```python
from build123d import *

# Parameters (mm, degrees)
F2_SIZE = 0.2


with BuildPart() as f1:
    # F0 (on Front) → F1 (revolve)
    with BuildSketch(Plane.XZ):
        Polygon((3.8, 27), (3.8, 0), (4.5, 0), (4.5, 14.8), (6.5, 14.8), (6.5, 21.4), (4.5, 21.4), (4.5, 27), align=None)
    revolve(axis=Axis((0, 0, 50), (0, 0, -1)))

    # F2
    f2_edges = [f1.edges().sort_by_distance(p)[0] for p in [
        (-4.5, 0, 0),
        (-6.5, 0, 14.8),
        (-6.5, 0, 21.4),
        (-4.5, 0, 27),
        (-3.8, 0, 27),
        (-3.8, 0, 0),
    ]]
    chamfer(f2_edges, length=F2_SIZE)


solid = f1.part
```
Part model, mm, in its own coordinate system. A direction names the side the tool comes from. Round coordinates to 2 decimals unless told otherwise and drop trailing zeros. Write each loop counter-clockwise with the first axis right and the second up, starting at its lowest first coordinate (ties: lowest second). Pieces come first, ordered by that corner, then holes. Notation, with made-up numbers: M -4,54 L 4,54 A13 ccw 4,62 Z; hole C -7,76.5 d10. An arc over 180 degrees is marked long. One line per question, with ' | ' between items.
(1) Saw through at C-C on z = 20.5. Write the cut outline in (x, y), then the cut area to 3 significant figures.
Answer key:
outline: C 0,0 d13; hole C 0,0 d7.6 | area: 87.4 mm^2
(2) Two-plate mould, pull along X, no slides. Class faces 1 (the face through (4, 3, 21.4)), 2 (the face through (-3.796, -0.167, 13.314)), 3 (the face through (-0.59, -4.46, 24.14)): released by +X, released by -X, zero draft, split by the parting line, or undercut.
Answer key:
face 1: zero draft | face 2: undercut | face 3: split by the parting line
(3) Saw through at A-A on y = 0. Write the cut outline in (x, z).
Answer key:
outline: M -6.5,15 L -6.3,14.8 L -4.5,14.8 L -4.5,0.2 L -4.3,0 L -4,0 L -3.8,0.2 L -3.8,26.8 L -4,27 L -4.3,27 L -4.5,26.8 L -4.5,21.4 L -6.3,21.4 L -6.5,21.2 Z; M 3.8,0.2 L 4,0 L 4.3,0 L 4.5,0.2 L 4.5,14.8 L 6.3,14.8 L 6.5,15 L 6.5,21.2 L 6.3,21.4 L 4.5,21.4 L 4.5,26.8 L 4.3,27 L 4,27 L 3.8,26.8 Z
(4) Probe line 1 along Y through (x, z) = (0, 8.25); line 2 along Y through (x, z) = (0, 17.25). List the from-to ranges inside material, lowest first.
Answer key:
line 1: y = -4.5 to -3.8, 3.8 to 4.5 | line 2: y = -6.5 to -3.8, 3.8 to 6.5
(5) 3-axis set-ups, long thin cutter, end or side, ignore diameter. For faces 4 (the face through (-5.158, 3.955, 18.143)), 5 (the face through (-4, 3, 14.8)): which of +Z, -Z, +X, -X, +Y, -Y reach the whole face in a straight line?
Answer key:
face 4: +Z, -Z | face 5: -Z
(6) Saw through at D-D on z = 3. Write the cut outline in (x, y), then the cut area to 3 significant figures.
Answer key:
outline: C 0,0 d9; hole C 0,0 d7.6 | area: 18.3 mm^2
(7) Pin check, flat tips, straight feed: pin 1 (6 mm diameter, centred on x = -1, z = 9.5, fed in from -Y); pin 2 (6 mm diameter, centred on x = 5, z = 14, fed in from -Y); pin 3 (4 mm diameter, centred on x = -1, z = 10.5, fed in from +Y); pin 4 (6.5 mm diameter, centred on x = 2, y = 3, fed in from +Z). Stop position of each tip, or through.
Answer key:
pin 1: stops at y = -4.5 | pin 2: stops at y = -6.13 | pin 3: stops at y = 4.5 | pin 4: stops at z = 27
